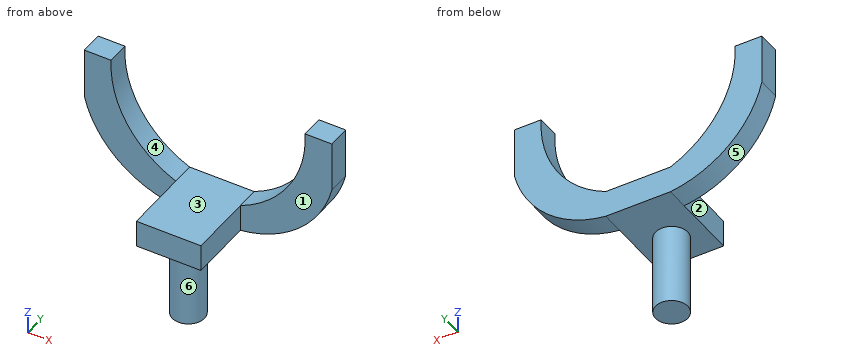
Autodesk Inventor part; units mm, degrees
ref_plane "YZ Plane" through (0, 0, 0) normal (1, 0, 0) x (0, 1, 0)
ref_plane "XZ Plane" through (0, 0, 0) normal (0, 1, 0) x (-1, 0, 0)
ref_plane "XY Plane" through (0, 0, 0) normal (0, 0, 1) x (1, 0, 0)
sketch "Sketch1" plane through (0, 0, 0) normal (0, 0, 1) x (1, 0, 0)
  circle A0 centre (0, 0) radius 6
  dimension "d0" = 12
extrude "Extrusion1" add sketch "Sketch1" along normal blind 30
sketch "Sketch2" plane through (0, 0, 30) normal (0, 0, 1) x (1, 0, 0)
  line L0 (0, 0) -> (12, 0)
  line L1 (12, 0) -> (12, 12)
  line L2 (12, 12) -> (0, 12)
  line L3 (0, 12) -> (0, 0)
  line L4 (0, 0) -> (12, 0)
  line L5 (12, 0) -> (12, -12)
  line L6 (12, -12) -> (0, -12)
  line L7 (0, -12) -> (0, 0)
  line L8 (0, 0) -> (-12, 0)
  line L9 (-12, 0) -> (-12, 12)
  line L10 (-12, 12) -> (0, 12)
  line L11 (0, 12) -> (0, 0)
  line L12 (-12, 0) -> (0, 0)
  line L13 (0, 0) -> (0, -12)
  line L14 (0, -12) -> (-12, -12)
  line L15 (-12, -12) -> (-12, 0)
  dimension "d3" = 12
  dimension "d4" = 12
  dimension "d5" = 12
  dimension "d6" = 12
extrude "Extrusion2" add sketch "Sketch2" along normal blind 10
sketch "Sketch3" plane through (-12, 12, 30) normal (0, 1, 0) x (1, 0, 0)
  line L0 (0, 0) -> (24, 0)
  line L1 (0, 0) -> (24, 0)
  line L2 (24, 0) -> (24, -48.9856)
  line L3 (24, -48.9856) -> (0, -48.9856)
  line L4 (0, -48.9856) -> (0, 0)
  line L5 (0, 0) -> (0, -10)
  line L6 (0, 0) -> (-24, 0)
  line L7 (-24, 0) -> (-24, -48.9856)
  line L8 (-24, -48.9856) -> (0, -48.9856)
  line L9 (0, -48.9856) -> (0, 0)
  arc A0 (0, -10) -> (-24, -48.9856) centre (15.934, -46.6893) ccw
  line L10 (24, 0) -> (24, -10)
  line L11 (24, 0) -> (48, 0)
  line L12 (48, 0) -> (48, -48.9856)
  line L13 (48, -48.9856) -> (24, -48.9856)
  line L14 (24, -48.9856) -> (24, 0)
  line L15 (0, -10) -> (24, -10)
  arc A1 (48, -48.9856) -> (24, -10) centre (8.066, -46.6893) ccw
  line L16 (-24, -48.9856) -> (-34, -48.9856)
  line L17 (-34, -48.9856) -> (-34, 0)
  line L18 (-34, 0) -> (-24, 0)
  line L19 (-24, 0) -> (-24, -48.9856)
  line L20 (48, 0) -> (58, 0)
  line L21 (58, 0) -> (58, -48.9856)
  line L22 (58, -48.9856) -> (48, -48.9856)
  line L23 (48, -48.9856) -> (48, 0)
  arc A2 (0, 0) -> (-34, -48.9856) centre (4.9068, -39.6979) ccw
  arc A3 (58, -48.9856) -> (24, 0) centre (19.0932, -39.6979) ccw
  point P0 (12, 30)
  point P1 (58, -30.4102)
  point P2 (-34, -30.4102)
  dimension "d9" = 24
  dimension "d10" = 24
  dimension "d11" = 40
  dimension "d12" = 24
  dimension "d13" = 40
  dimension "d14" = 10
  dimension "d15" = 10
  dimension "d16" = 40
  dimension "d17" = 40
extrude "Extrusion3" add sketch "Sketch3" along normal blind 8.4125 contours L0 L2 L15 L4 | L4 A0 L7 A2 | A3 L12 A1 L2 | L7 A0 L16 L17 A2 | A3 L21 L22 A1 L12
properties part number "End"
Check sheet for the modelled part. Datum: model origin and axes. Units: mm. Face numbers are marked on the shaded views. A direction names the side the tool comes from. Coordinates: 2 decimals unless noted, no trailing zeros. Loops run counter-clockwise (first coordinate to the right, second up) from the corner with the lowest first, then second, coordinate; pieces in that order, holes last. Notation, with made-up numbers: M -9.75,-13 L 39.25,-13 A12 cw 39.25,2 Z; hole C 47,42 d5. An arc over 180 degrees is marked long. Answer as a JSON object with one key per item and string values.
1. Sectioned sample at A-A on x = 0. Record the cut outline in (y, z).
Outcome:
{"outline": "M -12,30 L -6,30 L -6,0 L 6,0 L 6,30 L 20.41,30 L 20.41,40 L -12,40 Z"}
2. Release check for a two-part mould opening along X. For the marked faces 4, 5 and 6 record: pulls with the +X half, pulls with the -X half, needs draft (parallel to the pull), parting line crosses it, or undercut.
Outcome:
{"face 4": "undercut", "face 5": "pulls with the -X half", "face 6": "parting line crosses it"}
3. Sectioned sample at B-B on y = 0. Record the cut outline in (x, z).
Outcome:
{"outline": "M -12,30 L -6,30 L -6,0 L 6,0 L 6,30 L 12,30 L 12,40 L -12,40 Z"}
4. Depth check by flat-ended pin: P1, Ø8, axis at y = -1.5, z = 33.5, coming from the +X side; P2, Ø1.5, axis at x = 3.5, y = 6.5, coming from the -Z side; P3, Ø8, axis at x = -7.5, y = 7.5, coming from the +Z side; P4, Ø2, axis at y = 10, z = 62, coming from the -X side. Enter the tip coordinate at first touch or a pass-through.
Outcome:
{"P1": "x = 12", "P2": "z = 30", "P3": "z = 40", "P4": "through"}
5. Sectioned sample at D-D on z = 13.5. Record the cut outline in (x, y), and give its area (3 significant figures).
Outcome:
{"outline": "C 0,0 d12", "area": "113 mm²"}
6. Sectioned sample at C-C on z = 45.5. Record the cut outline in (x, y), and give its area (3 significant figures).
Outcome:
{"outline": "M -38.94,12 L -21.11,12 L -21.11,20.41 L -38.94,20.41 Z; M 21.11,12 L 38.94,12 L 38.94,20.41 L 21.11,20.41 Z", "area": "300 mm²"}
7. Access from +Z, -Z, +X, -X, +Y, -Y to the whole of each face (thin tool, end or side, straight path). Record for the marked faces 1, 2 and 3.
Outcome:
{"face 1": "+Z, -Z, +X, -Y", "face 2": "+Z, -Z, -X, -Y", "face 3": "+Z, +Y, -Y"}
8. Scan lines: L1, parallel to Y at x = 27.5, z = 51.5; L2, parallel to Z at x = 9.5, y = 1; L3, parallel to X at y = 13.5, z = 50.5. Record each from-to range of solid material in increasing order. Write a range as from..to.
Outcome:
{"L1": "12..20.41", "L2": "30..40", "L3": "-42.19..-26.3, 26.3..42.19"}
